For this review, take the finished solid that the model builds, in its own axes (mm). A direction names the side the tool comes from. Round coordinates to 2 decimals unless told otherwise and drop trailing zeros. Write each loop counter-clockwise with the first axis right and the second up, starting at its lowest first coordinate (ties: lowest second). Pieces come first, ordered by that corner, then holes. Notation, with made-up numbers: (-37, 85.25) - (-1, 85.25) arc R18 ccw to (-1, 107.25) - close; hole circle Ø10 at (12.25, 71). An arc over 180 degrees is marked (long way). One line per item, written item: value. Start each with the question number.
Q1. Add section A-A on y = 36. Write out the cut boundary in (x, z).
Q2. Add section B-B on y = -1. Write out the cut boundary in (x, z).
Q3. For probe 1 along Z at (x, y) = (0, 36); probe 2 along X at (y, z) = (19, 10) (1 decimal); probe 3 along Y at (x, z) = (-26.5, 21), list the stretches that pass through material, from the lowest coordinate up.
Q4. Clearance check with flat-ended pins moving along their axes: pin 1 Ø6 at (y, z) = (-5.5, 8.5) entering from -X (3 decimals); pin 2 Ø4 at (x, y) = (-12, 10.5) entering from -Z (3 decimals); pin 3 Ø4 at (x, z) = (1, -19) entering from +Y; pin 4 Ø0.8 at (x, z) = (-1, 4.5) entering from +Y. State where each tip first meets the part, or that it passes through.
Q5. Tool access review of faces 4 (the face through (0.806, 41.515, 2.879)), 5 (the face through (-29, -23.25, -10)), 6 (the face through (-1, 17.42, -18.69)): name each direction out of +Z, -Z, +X, -X, +Y, -Y from which nothing blocks a thin tool from reaching the whole face with its end or side.
Q6. Add section C-C on y = 17.5. Write out the cut boundary in (x, z), and give its area (3 significant figures).
Q7. Add section D-D on y = -28.5. Write out the cut boundary in (x, z), and give its area (3 significant figures).
Q8. Mouldability with a two-part tool opening along X and no side actions: class faces 1 (the face through (0.11, 28.21, 0.35)), 2 (the face through (0.231, 32.864, -5.245)), 3 (the face through (0, 37, 4.25)) as +X half, -X half, draft (parallel to the pull), parting line (faces both ways), or undercut.
```python
from build123d import *

# Parameters (mm, degrees)
SKETCH_1_R             = 35.8
EXTRUDE_1_DEPTH        = 23.25
HOLE_WIZARD_M4_1_D     = 3.3
HOLE_WIZARD_M4_1_DEPTH = 11.5
HOLE_WIZARD_M4_1_TIP   = 0.991420021
SKETCH_4_R             = 5.25
EXTRUDE_2_DEPTH        = 20
FILLET_1_R             = 0.5
SKETCH_5_W             = 9.627947462
SKETCH_5_H             = 2
CUT_EXTRUDE_1_DEPTH    = 12
HOLE_WIZARD_M5_1_D     = 4.2
HOLE_WIZARD_M5_1_DEPTH = 14
HOLE_WIZARD_M5_1_TIP   = 1.2618073
CHAMFER_1_SIZE         = 1
SKETCH_7_R             = 30
EXTRUDE_3_DEPTH        = 17
CHAMFER_2_SIZE         = 1
CHAMFER_3_SIZE         = 1
CHAMFER_3_SIZE2        = 3
SKETCH_8_R             = 1.5
CUT_EXTRUDE_2_DEPTH    = 69.965244933


with BuildPart() as part:
    # 草图1 → 凸台-拉伸1 (new, symmetric)
    with BuildSketch(Plane(origin=(0, 0, 0), x_dir=(1, 0, 0), z_dir=(0, 1, 0))):
        with Locations(Location((0, 0, 0), (0, 0, 90))):
            Circle(SKETCH_1_R)
    extrude(amount=EXTRUDE_1_DEPTH, both=True)

    # M4 螺纹孔1
    with Locations(Plane(origin=(0, 23.25, -20), x_dir=(0, 0, 1), z_dir=(0, 1, 0))):
        with Locations((0, 0), (30, -17.320508076), (30, 17.320508076)):
            Hole(HOLE_WIZARD_M4_1_D / 2, depth=HOLE_WIZARD_M4_1_DEPTH)
            with Locations((0, 0, -(HOLE_WIZARD_M4_1_DEPTH + HOLE_WIZARD_M4_1_TIP / 2))):  # 118° drill point
                Cone(0, HOLE_WIZARD_M4_1_D / 2, HOLE_WIZARD_M4_1_TIP, mode=Mode.SUBTRACT)

    # 草图4 → 凸台-拉伸2 (add)
    with BuildSketch(Plane(origin=(0, 23.25, 0), x_dir=(1, 0, 0), z_dir=(0, 1, 0))):
        with Locations(Location((0, 0, 0), (0, 0, 270))):
            Circle(SKETCH_4_R)
    extrude(amount=EXTRUDE_2_DEPTH)

    # 圆角1
    fillet_1_edges = [part.edges().sort_by_distance(p)[0] for p in [
        (0, 43.25, -5.25),
    ]]
    fillet(fillet_1_edges, radius=FILLET_1_R)

    # 草图5 → 切除-拉伸1 (cut)
    with BuildSketch(Plane(origin=(0, 43.25, 0), x_dir=(1, 0, 0), z_dir=(0, 1, 0))):
        with Locations((0, -5.25)):
            Rectangle(SKETCH_5_W, SKETCH_5_H)
    extrude(amount=-CUT_EXTRUDE_1_DEPTH, mode=Mode.SUBTRACT)

    # M5 螺纹孔1
    with Locations(Plane.ZX.offset(43.25)):
        with Locations((0, 0)):
            Hole(HOLE_WIZARD_M5_1_D / 2, depth=HOLE_WIZARD_M5_1_DEPTH)
            with Locations((0, 0, -(HOLE_WIZARD_M5_1_DEPTH + HOLE_WIZARD_M5_1_TIP / 2))):  # 118° drill point
                Cone(0, HOLE_WIZARD_M5_1_D / 2, HOLE_WIZARD_M5_1_TIP, mode=Mode.SUBTRACT)

    # 倒角1
    chamfer_1_edges = [part.edges().sort_by_distance(p)[0] for p in [
        (0, 23.25, 35.8),
    ]]
    chamfer(chamfer_1_edges, length=CHAMFER_1_SIZE)

    # 草图7 → 凸台-拉伸3 (add)
    with BuildSketch(Plane.XZ.offset(23.25)):
        with Locations(Location((0, 0, 0), (0, 0, 90))):
            Circle(SKETCH_7_R)
    extrude(amount=EXTRUDE_3_DEPTH)

    # 倒角2
    chamfer_2_edges = [part.edges().sort_by_distance(p)[0] for p in [
        (0, -23.25, 35.8),
    ]]
    chamfer(chamfer_2_edges, length=CHAMFER_2_SIZE)

    # 倒角3
    chamfer_3_edges = [part.edges().sort_by_distance(p)[0] for p in [
        (0, -40.25, -30),
    ]]
    chamfer_3_side = [part.faces().sort_by_distance(p)[0] for p in [
        (0, -31.75, -30),
    ]]
    chamfer(chamfer_3_edges, length=CHAMFER_3_SIZE, length2=CHAMFER_3_SIZE2, reference=chamfer_3_side[0])

    # 草图8 → 切除-拉伸2 (cut, through all)
    with BuildSketch(Plane.XY.offset(4.25)):
        with Locations((0, 40.25)):
            Circle(SKETCH_8_R)
    extrude(amount=-CUT_EXTRUDE_2_DEPTH, mode=Mode.SUBTRACT)


solid = part.part
```
Result set:
1. outline: (-3.08, 4.25) arc R5.25 ccw (long way) to (3.08, 4.25) - close; hole circle Ø4.2 at (0, 0)
2. outline: circle Ø71.6 at (0, 0)
3. probe 1: z = -5.25 to -2.1, 2.1 to 4.25
3. probe 2: x = -34.4 to -19, -15.7 to 15.7, 19 to 34.4
3. probe 3: y = -23.25 to 23.25
4. pin 1: stops at x = -35.375
4. pin 2: stops at z = -34.375
4. pin 3: stops at y = 23.25
4. pin 4: stops at y = 43.25
5. face 4: +Z, -Z
5. face 5: -Y
5. face 6: +Y
6. outline: circle Ø71.6 at (0, 0); hole circle Ø3.3 at (-17.32, 10); hole circle Ø3.3 at (0, -20); hole circle Ø3.3 at (17.32, 10)
6. area: 4,000 mm^2
7. outline: circle Ø60 at (0, 0)
7. area: 2,830 mm^2
8. face 1: undercut
8. face 2: parting line
8. face 3: draft
